Here's the drawing with two shaded views (mm, measured from the low corner). I have some questions. Coordinates: 2 decimals unless noted, no trailing zeros. Order: outer loops, then holes, each group sorted by start corner. A loop starts at its lowest first (then second) coordinate and runs counter-clockwise, first axis right, second up. Notation, with made-up numbers: (78.25, 76) - (112.25, 76) arc R18 cw to (112.25, 91) - close; hole circle Ø1 at (65.25, -15.75). An arc over 180 degrees is marked (long way). Answer as a JSON object with one key per item and string values. Group by question number.
(1) Please list where these lines run through material, in increasing order: probe 1 along Z at (x, y) = (94.5, 2.1); probe 2 along X at (y, z) = (1.55, 77); probe 3 along Z at (x, y) = (16, 2.05).
(2) Will this pin go through, and if not, where does the flat tip stop? P1, Ø1.5, axis at y = 1.5, z = 120, coming from the +X side.
(3) Imagine slicing it at B-B, the plane z = 51.5. Write out the boundary of the cut face in (x, y).
(4) Imagine slicing it at A-A, the plane y = 2.1. Write out the boundary of the cut face in (x, z), and give its area (3 significant figures).
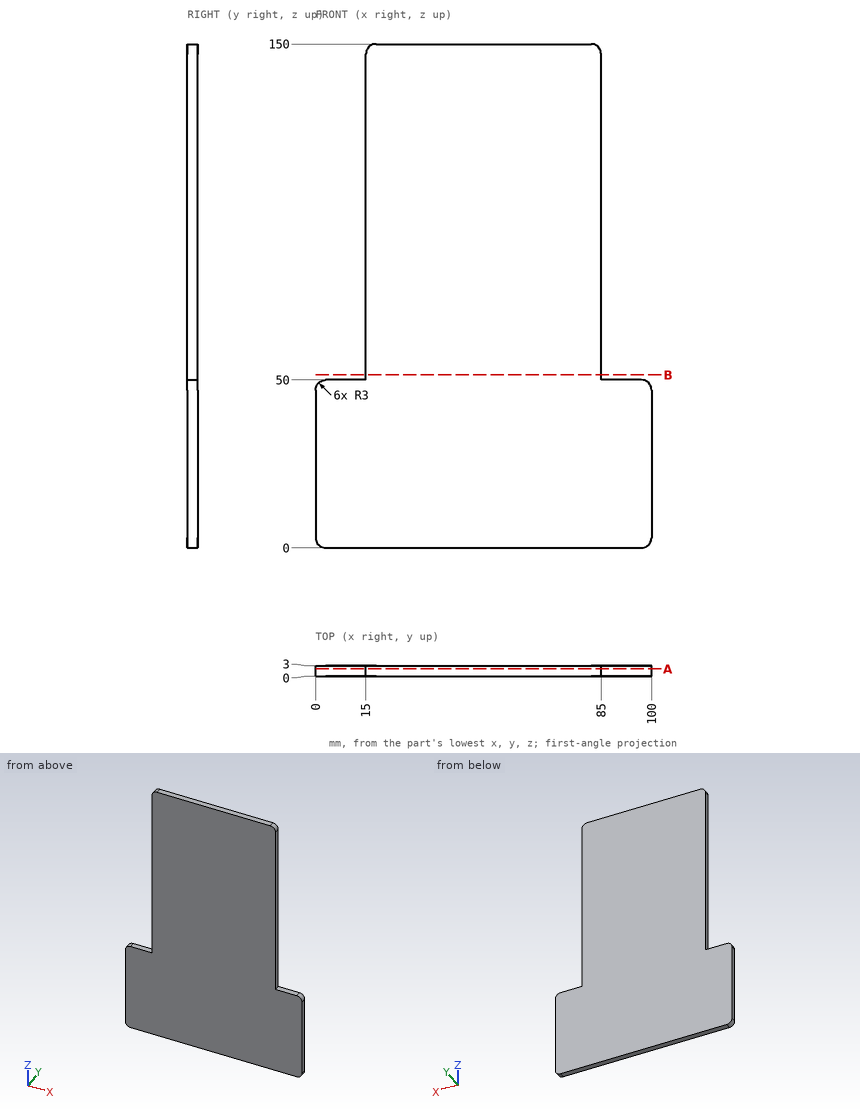
Result set:
{
 "1": {"probe 1": "z = 0 to 50", "probe 2": "x = 15 to 85", "probe 3": "z = 0 to 149.24"},
 "2": {"P1": "stops at x = 85"},
 "3": {"outline": "(15, 0) - (85, 0) - (85, 3) - (15, 3) - close"},
 "4": {"outline": "(0, 3) arc R3 ccw to (3, 0) - (97, 0) arc R3 ccw to (100, 3) - (100, 47) arc R3 ccw to (97, 50) - (85, 50) - (85, 147) arc R3 ccw to (82, 150) - (18, 150) arc R3 ccw to (15, 147) - (15, 50) - (3, 50) arc R3 ccw to (0, 47) - close", "area": "12,000 mm^2"}
}
